Input: part model. Units: mm. Frame: model coordinates. A direction names the side the tool comes from. Give positions to 0.01 mm unless a question says otherwise; leave off trailing zeros. Loops run counter-clockwise (first coordinate to the right, second up) from the corner with the lowest first, then second, coordinate; pieces in that order, holes last. Notation, with made-up numbers: M 40.25,-17.75 L 44.25,-17.75 A15 cw 44.25,-8.75 Z; hole C -21.5,20.25 d4. An arc over 180 degrees is marked long. Use CSV: the item, a comma, the result in double quotes. Start each with the question number.
Q1. Reachability of faces 4 (the flat face through (63, 0, -7)), 5 (the flat face through (64, 0, 5)), 6 (the flat face through (81, -4, 3.25)), 7 (the flat face through (65, 0, 2)) from +Z, -Z, +X, -X, +Y, -Y: full face, straight path, thin tool, end or side. Return the list, or none.
Q2. Section A-A, the plane x = 76.75. Output: boundary loops of the cut face in (y, z).
Q3. Material intervals for line 1 along Z through (x, y) = (82.75, 2); line 2 along Y through (x, z) = (87, 1); line 3 along X through (y, z) = (-1, -12.5), sorted ascending.
Q4. Pull-direction query (Z, two-part tool) for faces 1 (the flat face through (77, 3, 0)), 2 (the flat face through (81, -4, 6.75)), 3 (the flat face through (90, 4, 2)); classes: released by +Z, released by -Z, zero draft, split by the parting line, or undercut.
Q5. Section B-B, the plane z = 8.5. Output: boundary loops of the cut face in (x, y), plus the area to 3 significant figures.
Q6. Pin query (flat end, axial travel): pin 1 (4 mm diameter, centred on y = 0, z = 2, fed in from +X); pin 2 (1.5 mm diameter, centred on x = 80, y = -4, fed in from -Z); pin 3 (1.5 mm diameter, centred on x = 65.5, y = 4, fed in from +Z). Return the tip coordinate at first contact, or that it passes through.
Q7. Section D-D, the plane z = -7.25. Output: boundary loops of the cut face in (x, y).
Q8. Section C-C, the plane z = 1.5. Output: boundary loops of the cut face in (x, y).
from build123d import *

# Parameters (mm, degrees)
SALIENTE_EXTRUIR1_DEPTH = 10
CORTAR_EXTRUIR1_DEPTH   = 92.569427212
CROQUIS3_W              = 3
CROQUIS3_H              = 13.6
SALIENTE_EXTRUIR2_DEPTH = 15
CHAFL_N1_SIZE           = 10
CHAFL_N1_SIZE2          = 2.679491924
REDONDEO1_R             = 3
CROQUIS4_W              = 167.371615842
CROQUIS4_H              = 49.121487425
CORTAR_EXTRUIR2_DEPTH   = 93.249444443


with BuildPart() as part:
    # Croquis1 → Saliente-Extruir1 (new body)
    with BuildSketch(Plane.XY):
        Polygon((-90, -6.8), (-90, -1.8), (-65, -1.8), (-65, 1.8), (-90, 1.8), (-90, 6.8), (90, 6.8), (90, 1.8), (65, 1.8), (65, -1.8), (90, -1.8), (90, -6.8), align=None)
    extrude(amount=SALIENTE_EXTRUIR1_DEPTH)

    # Croquis2 → Cortar-Extruir1 (cut, through all)
    with BuildSketch(Plane(origin=(0, 6.8, 0), x_dir=(1, 0, 0), z_dir=(0, 1, 0))):
        with BuildLine():
            Line((-76.25, -3.25), (-86.25, -3.25))
            ThreePointArc((-86.25, -3.25), (-88, -5), (-86.25, -6.75))
            Line((-86.25, -6.75), (-76.25, -6.75))
            ThreePointArc((-76.25, -6.75), (-74.5, -5), (-76.25, -3.25))
        make_face()
        with BuildLine():
            ThreePointArc((-90, -5), (-88.958333333, -1.875), (-86.25, 0))
            Line((-86.25, 0), (-90, 0))
            Line((-90, 0), (-90, -5))
        make_face()
        with BuildLine():
            Line((86.25, -10), (90, -10))
            Line((90, -10), (90, -5))
            ThreePointArc((90, -5), (88.958333333, -8.125), (86.25, -10))
        make_face()
        with BuildLine():
            Line((76.25, -6.75), (86.25, -6.75))
            ThreePointArc((86.25, -6.75), (88, -5), (86.25, -3.25))
            Line((86.25, -3.25), (76.25, -3.25))
            ThreePointArc((76.25, -3.25), (74.5, -5), (76.25, -6.75))
        make_face()
        with BuildLine():
            Line((71.25, -5), (-71.25, -5))
            ThreePointArc((-71.25, -5), (-72.847588014, -8.335363746), (-76.15, -10))
            Line((-76.15, -10), (76.15, -10))
            ThreePointArc((76.15, -10), (72.847588014, -8.335363746), (71.25, -5))
        make_face()
    extrude(amount=-CORTAR_EXTRUIR1_DEPTH, mode=Mode.SUBTRACT)

    # Croquis3 → Saliente-Extruir2 (add)
    with BuildSketch(Plane(origin=(0, 0, 0), x_dir=(-1, 0, 0), z_dir=(0, 0, -1))):
        with Locations((-61.5, 0)):
            Rectangle(CROQUIS3_W, CROQUIS3_H)
        with Locations((61.5, 0)):
            Rectangle(CROQUIS3_W, CROQUIS3_H)
    extrude(amount=SALIENTE_EXTRUIR2_DEPTH)

    # Chaflán1
    chafl_n1_edges = [part.edges().sort_by_distance(p)[0] for p in [
        (0, -6.8, 0),
    ]]
    chafl_n1_side = [part.faces().sort_by_distance(p)[0] for p in [
        (0, 0, 0),
    ]]
    chamfer(chafl_n1_edges, length=CHAFL_N1_SIZE, length2=CHAFL_N1_SIZE2, reference=chafl_n1_side[0])

    # Redondeo1
    redondeo1_edges = [part.edges().sort_by_distance(p)[0] for p in [
        (61.5, 6.8, -15),
        (61.5, -6.8, -15),
        (-61.5, 6.8, -15),
        (-61.5, -6.8, -15),
    ]]
    fillet(redondeo1_edges, radius=REDONDEO1_R)

    # Croquis4 → Cortar-Extruir2 (cut, through all)
    with BuildSketch(Plane(origin=(0, -6.8, 0), x_dir=(-1, 0, 0), z_dir=(0, -1, 0))):
        with Locations((23.685807921, 0.224960459)):
            Rectangle(CROQUIS4_W, CROQUIS4_H)
    extrude(amount=-CORTAR_EXTRUIR2_DEPTH, mode=Mode.SUBTRACT)


solid = part.part
A:
1,face 4,"-Z, +X, +Y, -Y"
1,face 5,"+Z, -X, +Y, -Y"
1,face 6,"+Y, -Y"
1,face 7,"+Z, -Z, +X"
2,outline,"M -6.8,0 L -1.8,0 L -1.8,3.25 L -6.8,3.25 Z; M -6.8,6.75 L -1.8,6.75 L -1.8,10 L -6.8,10 Z; M 1.8,0 L 6.8,0 L 6.8,3.25 L 1.8,3.25 Z; M 1.8,6.75 L 6.8,6.75 L 6.8,10 L 1.8,10 Z"
3,line 1,"0 to 3.25, 6.75 to 10"
3,line 2,"-6.8 to -1.8, 1.8 to 6.8"
3,line 3,"60 to 63"
4,face 1,"released by -Z"
4,face 2,"undercut"
4,face 3,"zero draft"
5,outline,"M 73.02,-6.8 L 88.65,-6.8 L 88.65,-1.8 L 73.02,-1.8 Z; M 73.02,1.8 L 88.65,1.8 L 88.65,6.8 L 73.02,6.8 Z"
5,area,"156 mm^2"
6,pin 1,"x = 90"
6,pin 2,"z = 0"
6,pin 3,"z = 5"
7,outline,"M 60,-6.8 L 63,-6.8 L 63,6.8 L 60,6.8 Z"
8,outline,"M 60,-6.8 L 90,-6.8 L 90,-1.8 L 65,-1.8 L 65,1.8 L 90,1.8 L 90,6.8 L 60,6.8 Z"
